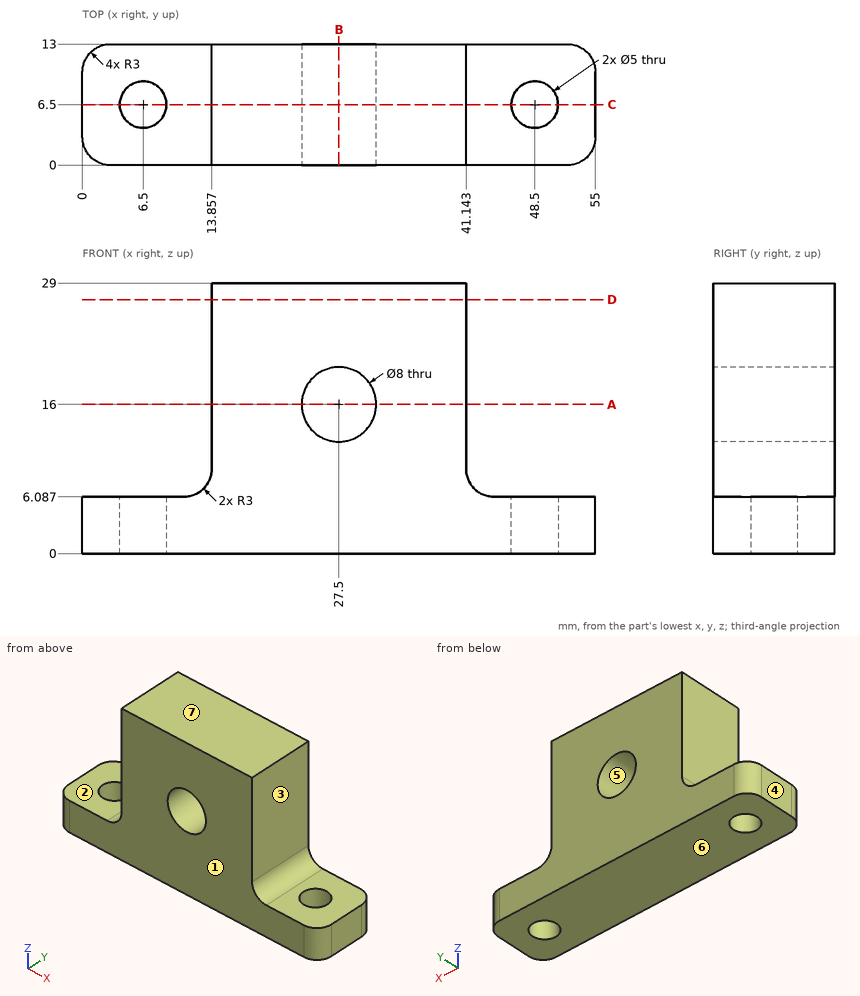
Geometry: see drawing. Coordinates: mm, zero at the bounding-box minimum. A direction names the side the tool comes from. Round coordinates to 2 decimals unless told otherwise and drop trailing zeros. Write each loop counter-clockwise with the first axis right and the second up, starting at its lowest first coordinate (ties: lowest second). Pieces come first, ordered by that corner, then holes. Notation, with made-up numbers: M 63,-8 L 71,-8 A17 ccw 71,21 Z; hole C 42,65 d6. An arc over 180 degrees is marked long. Answer in a Markdown table with one row per item. Add a question column.
(1) Ray query, L1, parallel to Y at x = 48.5, z = 4.5; L2, parallel to Z at x = 27.5, y = 3; L3, parallel to Z at x = 10, y = 3.5. Return the intervals inside material, ascending.
(2) Reachability of the marked faces 1, 2 and 3 from +Z, -Z, +X, -X, +Y, -Y: full face, straight path, thin tool, end or side. Return the list, or none.
(3) Cut plane A-A, the plane z = 16. Return the cut outline in (x, y).
(4) Draft query along Z for the marked faces 4, 5, 6 and 7. Return one class per face: pulls with the +Z half, pulls with the -Z half, needs draft (parallel to the pull), parting line crosses it, or undercut.
(5) Cut plane D-D, the plane z = 27.25. Return the cut outline in (x, y).
(6) Contact query for flat-ended pins moving along their axis: pin 1 (1.5 mm diameter, centred on y = 5.5, z = 17.5, fed in from -X); pin 2 (5.5 mm diameter, centred on x = 6, y = 9.5, fed in from +Z). Output: stop coordinate, or through.
(7) Cut plane C-C, the plane y = 6.5. Return the cut outline in (x, z).
(8) Cut plane B-B, the plane x = 27.5. Return the cut outline in (y, z).
Established:
| question | item | result |
|---|---|---|
| 1 | L1 | 0 to 4, 9 to 13 |
| 1 | L2 | 0 to 12, 20 to 29 |
| 1 | L3 | 0 to 6.09 |
| 2 | face 1 | +Z, -Z, +X, -X, -Y |
| 2 | face 2 | +Z, -X, +Y, -Y |
| 2 | face 3 | +Z, +X, +Y, -Y |
| 3 | outline | M 13.86,0 L 23.5,0 L 23.5,13 L 13.86,13 Z; M 31.5,0 L 41.14,0 L 41.14,13 L 31.5,13 Z |
| 4 | face 4 | needs draft |
| 4 | face 5 | undercut |
| 4 | face 6 | pulls with the -Z half |
| 4 | face 7 | pulls with the +Z half |
| 5 | outline | M 13.86,0 L 41.14,0 L 41.14,13 L 13.86,13 Z |
| 6 | pin 1 | x = 13.86 |
| 6 | pin 2 | z = 6.09 |
| 7 | outline | M 0,0 L 4,0 L 4,6.09 L 0,6.09 Z; M 9,0 L 46,0 L 46,6.09 L 44.14,6.09 A3 cw 41.14,9.09 L 41.14,29 L 13.86,29 L 13.86,9.09 A3 cw 10.86,6.09 L 9,6.09 Z; M 51,0 L 55,0 L 55,6.09 L 51,6.09 Z; hole C 27.5,16 d8 |
| 8 | outline | M 0,0 L 13,0 L 13,12 L 0,12 Z; M 0,20 L 13,20 L 13,29 L 0,29 Z |
